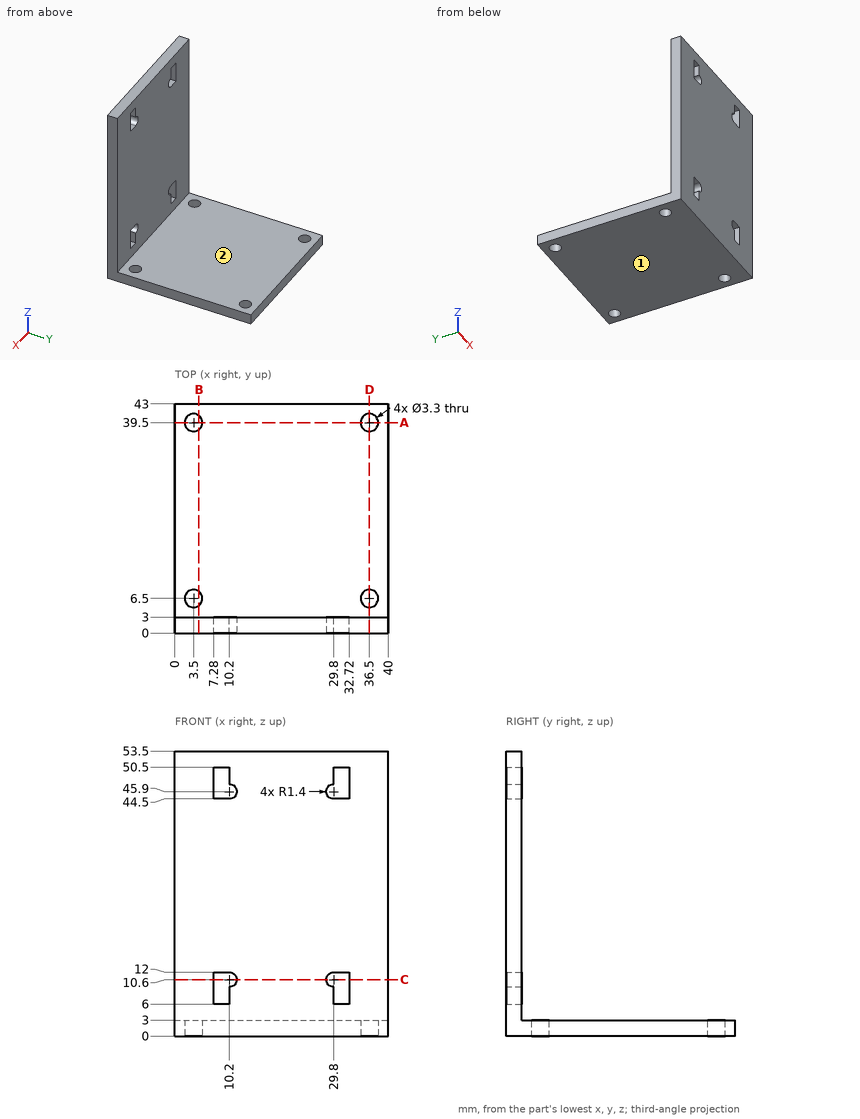
The drawing under review shows one solid part. Ordinate dimensions are in mm from its lowest x, y, z. A direction names the side the tool comes from. Coordinates: 2 decimals unless noted, no trailing zeros. Loops run counter-clockwise (first coordinate to the right, second up) from the corner with the lowest first, then second, coordinate; pieces in that order, holes last. Notation, with made-up numbers: (84, 31.5) -> (133, 31.5) arc R15 ccw to (133, 57.5) -> close; hole circle Ø11 at (54.5, 58). An arc over 180 degrees is marked (long way). Answer as a JSON object with one key per item and string values.
Q1. Take a section at A-A on y = 39.5. Give the boundary of the cut face in (x, z), plus the area to 3 significant figures.
Answer block:
{"outline": "(0, 0) -> (1.85, 0) -> (1.85, 3) -> (0, 3) -> close; (5.15, 0) -> (34.85, 0) -> (34.85, 3) -> (5.15, 3) -> close; (38.15, 0) -> (40, 0) -> (40, 3) -> (38.15, 3) -> close", "area": "100 mm^2"}
Q2. To check wall thickness, follow L1, parallel to Y at x = 3.5, z = 2; L2, parallel to Z at x = 34.5, y = 5.5; L3, parallel to X at y = 39, z = 1. State the ranges of each line that lie inside material, in increasing order.
Answer block:
{"L1": "y = 0 to 4.85, 8.15 to 37.85, 41.15 to 43", "L2": "z = 0 to 3", "L3": "x = 0 to 1.93, 5.07 to 34.93, 38.07 to 40"}
Q3. Tool access review of the marked faces 1 and 2: name each direction out of +Z, -Z, +X, -X, +Y, -Y from which nothing blocks a thin tool from reaching the whole face with its end or side.
Answer block:
{"face 1": "-Z, +X, -X, +Y, -Y", "face 2": "+Z, +X, -X, +Y"}
Q4. Take a section at C-C on z = 10.6. Give the boundary of the cut face in (x, y).
Answer block:
{"outline": "(0, 0) -> (7.28, 0) -> (7.28, 3) -> (0, 3) -> close; (11.6, 0) -> (28.4, 0) -> (28.4, 3) -> (11.6, 3) -> close; (32.72, 0) -> (40, 0) -> (40, 3) -> (32.72, 3) -> close"}
Q5. Take a section at D-D on x = 36.5. Give the boundary of the cut face in (y, z), plus the area to 3 significant figures.
Answer block:
{"outline": "(0, 0) -> (4.85, 0) -> (4.85, 3) -> (3, 3) -> (3, 53.5) -> (0, 53.5) -> close; (8.15, 0) -> (37.85, 0) -> (37.85, 3) -> (8.15, 3) -> close; (41.15, 0) -> (43, 0) -> (43, 3) -> (41.15, 3) -> close", "area": "261 mm^2"}
Q6. Take a section at B-B on x = 4.5. Give the boundary of the cut face in (y, z), plus the area to 3 significant figures.
Answer block:
{"outline": "(0, 0) -> (5.19, 0) -> (5.19, 3) -> (3, 3) -> (3, 53.5) -> (0, 53.5) -> close; (7.81, 0) -> (38.19, 0) -> (38.19, 3) -> (7.81, 3) -> close; (40.81, 0) -> (43, 0) -> (43, 3) -> (40.81, 3) -> close", "area": "265 mm^2"}
Q7. Clearance check with flat-ended pins moving along their axes: pin 1 Ø4.5 at (x, y) = (3.5, 39.5) entering from +Z; pin 2 Ø2 at (x, y) = (36.5, 39.5) entering from -Z; pin 3 Ø8 at (x, z) = (8.5, 48) entering from +Y; pin 4 Ø5 at (x, z) = (16, 44.5) entering from -Y. State where each tip first meets the part, or that it passes through.
Answer block:
{"pin 1": "stops at z = 3", "pin 2": "passes through", "pin 3": "stops at y = 3", "pin 4": "stops at y = 0"}
